```python
from build123d import *

# Parameters (mm, degrees)
BOSS_EXTRUDE1_DEPTH = 5
CUT_EXTRUDE1_DEPTH  = 5


with BuildPart() as part:
    # Sketch1 → Boss-Extrude1 (new body)
    with BuildSketch(Plane.XY):
        Polygon((-5.27676951, 0), (4.72323049, 0), (4.72323049, 5), (14.72323049, 5), (14.72323049, 49), (-15.27676951, 49), (-15.27676951, 5), (-5.27676951, 5), align=None)
    extrude(amount=BOSS_EXTRUDE1_DEPTH)

    # Sketch2 → Cut-Extrude1 (cut)
    with BuildSketch(Plane(origin=(0, 0, 0), x_dir=(-1, 0, 0), z_dir=(0, 0, -1))):
        Polygon((-1.472855596, 34.6), (2.927144404, 34.6), (2.927144404, 42.7), (4.427144404, 42.7), (4.427144404, 46), (2.927144404, 46), (2.927144404, 49), (-1.472855596, 49), (-1.472855596, 46), (-2.972855596, 46), (-2.972855596, 42.7), (-1.472855596, 42.7), align=None)
    extrude(amount=-CUT_EXTRUDE1_DEPTH, mode=Mode.SUBTRACT)


solid = part.part
```
Geometry: final body of the model. Coordinates: model frame, mm. A direction names the side the tool comes from. Round coordinates to 2 decimals unless told otherwise and drop trailing zeros. Loops run counter-clockwise (first coordinate to the right, second up) from the corner with the lowest first, then second, coordinate; pieces in that order, holes last. Notation, with made-up numbers: (76, 27) -> (123, 27) arc R8 cw to (123, 39) -> close; hole circle Ø6 at (89, 60). An arc over 180 degrees is marked (long way). Write each question's results on one line, items separated by ' | '.
Item 1: Cut plane C-C on x = -11.5. Return the cut outline in (y, z).
Answers below:
outline: (5, 0) -> (49, 0) -> (49, 5) -> (5, 5) -> close
Item 2: Cut plane D-D on y = 3. Return the cut outline in (x, z), and give its area (3 significant figures).
Answers below:
outline: (-5.28, 0) -> (4.72, 0) -> (4.72, 5) -> (-5.28, 5) -> close | area: 50.0 mm²
Item 3: Cut plane A-A on y = 43.5. Return the cut outline in (x, z), and give its area (3 significant figures).
Answers below:
outline: (-15.28, 0) -> (-4.43, 0) -> (-4.43, 5) -> (-15.28, 5) -> close; (2.97, 0) -> (14.72, 0) -> (14.72, 5) -> (2.97, 5) -> close | area: 113 mm²
Item 4: Cut plane B-B on z = 1. Return the cut outline in (x, y).
Answers below:
outline: (-15.28, 5) -> (-5.28, 5) -> (-5.28, 0) -> (4.72, 0) -> (4.72, 5) -> (14.72, 5) -> (14.72, 49) -> (1.47, 49) -> (1.47, 46) -> (2.97, 46) -> (2.97, 42.7) -> (1.47, 42.7) -> (1.47, 34.6) -> (-2.93, 34.6) -> (-2.93, 42.7) -> (-4.43, 42.7) -> (-4.43, 46) -> (-2.93, 46) -> (-2.93, 49) -> (-15.28, 49) -> close
Item 5: Pin query (flat end, axial travel): pin 1 Ø2.5 at (y, z) = (3, 3) entering from -X; pin 2 Ø1.5 at (x, z) = (-9.5, 3.5) entering from -Y; pin 3 Ø1.3 at (x, z) = (-1, 3.5) entering from +Y. Return the tip coordinate at first contact, or that it passes through.
Answers below:
pin 1: stops at x = -5.28 | pin 2: stops at y = 5 | pin 3: stops at y = 34.6
Item 6: Pull-direction query (X, two-part tool) for faces 6 (the face through (2, 46, 2)), 7 (the face through (-9, 49, 2)), 8 (the face through (4.723, 2, 2)); classes: pulls with the +X half, pulls with the -X half, needs draft (parallel to the pull), parting line crosses it, or undercut.
Answers below:
face 6: undercut | face 7: needs draft | face 8: pulls with the +X half
Item 7: Set-up query: faces 1 (the face through (-1, 34.6, 2)), 2 (the face through (0, 0, 2)), 3 (the face through (10, 5, 2)), 4 (the face through (-4, 46, 2)), 5 (the face through (-5.277, 3, 2)). Return all of +Z, -Z, +X, -X, +Y, -Y with unobstructed straight access to the full face (end or side cutting, diameter ignored); none if empty.
Answers below:
face 1: +Z, -Z, +Y | face 2: +Z, -Z, +X, -X, -Y | face 3: +Z, -Z, +X, -Y | face 4: +Z, -Z | face 5: +Z, -Z, -X, -Y
Item 8: Line query: probe 1 along X at (y, z) = (45.5, 3.9); probe 2 along X at (y, z) = (39, 3.6); probe 3 along Y at (x, z) = (2, 1.55). Output: solid intervals per line, ascending. Write a range as [from, to].
Answers below:
probe 1: x = [-15.28, -4.43], [2.97, 14.72] | probe 2: x = [-15.28, -2.93], [1.47, 14.72] | probe 3: y = [0, 42.7], [46, 49]
